from build123d import *

# Parameters (mm, degrees)
F1_DEPTH = 26
F3_DEPTH = 7
F4_R     = 5
F5_R     = 2.5


with BuildPart() as f1:
    # F0 (on Top) → F1 (new body)
    with BuildSketch(Plane.XY):
        Polygon((0, 30), (0, 0), (4, 0), (4, 26), (9.5, 26), (9.5, 0), (13.5, 0), (13.5, 15), (40.5, 20), (40.5, 120), (30.5, 120), (-5, 120), (-5, 110), (30.5, 110), (30.5, 30), align=None)
        with BuildLine():
            Line((4, 0), (0, 0))
            ThreePointArc((0, 0), (2, -2), (4, 0))
        make_face()
        with BuildLine():
            ThreePointArc((-5, 120), (-10, 115), (-5, 110))
            Line((-5, 110), (-5, 120))
        make_face()
        with BuildLine():
            Line((13.5, 0), (9.5, 0))
            ThreePointArc((9.5, 0), (11.5, -2), (13.5, 0))
        make_face()
    extrude(amount=F1_DEPTH)

    # F2 (on face) → F3 (cut)
    with BuildSketch(Plane(origin=(0, 0, 0), x_dir=(1, 0, 0), z_dir=(0, 0, -1))):
        with BuildLine():
            Line((13.5, -30), (30.5, -30))
            Line((30.5, -30), (30.5, -110))
            Line((30.5, -110), (-5, -110))
            ThreePointArc((-5, -110), (-10, -115), (-5, -120))
            Line((-5, -120), (13.5, -120))
            Line((13.5, -120), (40.5, -120))
            Line((40.5, -120), (40.5, -20))
            Line((40.5, -20), (13.5, -15))
            Line((13.5, -15), (13.5, -30))
        make_face()
    extrude(amount=-F3_DEPTH, mode=Mode.SUBTRACT)

    # F4
    f4_edges = [f1.edges().sort_by_distance(p)[0] for p in [
        (40.5, 120, 16.5),
        (30.5, 110, 16.5),
        (30.5, 30, 16.5),
        (40.5, 20, 16.5),
    ]]
    fillet(f4_edges, radius=F4_R)

    # F5
    f5_edges = [f1.edges().sort_by_distance(p)[0] for p in [
        (0, 30, 13),
        (4, 26, 13),
        (9.5, 26, 13),
        (13.5, 15, 16.5),
        (13.5, 30, 3.5),
    ]]
    fillet(f5_edges, radius=F5_R)


solid = f1.part
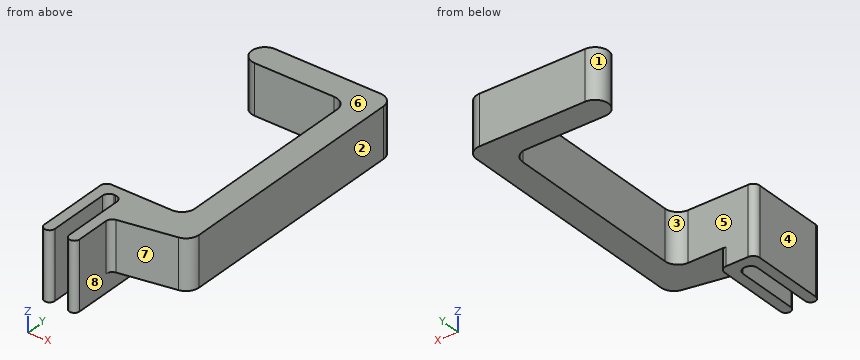
Input: part model. Units: mm. Frame: model coordinates. Face numbers are marked on the shaded views. A direction names the side the tool comes from. Coordinates: 2 decimals unless noted, no trailing zeros. Loops run counter-clockwise (first coordinate to the right, second up) from the corner with the lowest first, then second, coordinate; pieces in that order, holes last.
(1) Section C-C on x = 20.5. Return the cut outline in (y, z), then the cut area to 3 significant figures.
(2) Section D-D on y = 59.5. Return the cut outline in (x, z), then the cut area to 3 significant figures.
(3) First-contact query: pin 1 Ø12 at (y, z) = (17, 14) entering from +X; pin 2 Ø9.5 at (y, z) = (74, 14) entering from -X; pin 3 Ø4 at (x, z) = (34, 8.5) entering from -Y. Flat tips, straight axial feed; report the tip coordinate or a pass-through.
(4) Section B-B on z = 11.5. Return the cut outline in (x, y), then the cut area to 3 significant figures.
(5) Set-up query: the marked faces 4, 5, 6, 7 and 8. Return all of +Z, -Z, +X, -X, +Y, -Y with unobstructed straight access to the full face (end or side cutting, diameter ignored); none if empty.
(6) Pull-direction query (Y, two-part tool) for the marked faces 1, 2 and 3; classes: released by +Y, released by -Y, zero draft, split by the parting line, or undercut.
(7) Section A-A on y = 8. Return the cut outline in (x, z), then the cut area to 3 significant figures.
(8) Material intervals for probe 1 along X at (y, z) = (6, 25); probe 2 along Z at (x, y) = (33, 94); probe 3 along Y at (x, z) = (18, 17.5), sorted ascending.
Data:
1. outline: (16.3, 7) - (30, 7) - (30, 26) - (16.3, 26) - close; (110, 7) - (120, 7) - (120, 26) - (110, 26) - close
1. area: 450 mm2
2. outline: (30.5, 7) - (40.5, 7) - (40.5, 26) - (30.5, 26) - close
2. area: 190 mm2
3. pin 1: stops at x = 40.36
3. pin 2: stops at x = 30.5
3. pin 3: stops at y = 18.43
4. outline: (-5, 110) - (25.5, 110) arc R5 cw to (30.5, 105) - (30.5, 35) arc R5 cw to (25.5, 30) - (2.5, 30) arc R2.5 ccw to (0, 27.5) - (0, 0) arc R2 ccw to (4, 0) - (4, 23.5) arc R2.5 cw to (6.5, 26) - (7, 26) arc R2.5 cw to (9.5, 23.5) - (9.5, 0) arc R2 ccw to (13.5, 0) - (13.5, 12.92) arc R2.5 cw to (15.54, 15.38) - (36.41, 19.24) arc R5 ccw to (40.5, 24.16) - (40.5, 115) arc R5 ccw to (35.5, 120) - (-5, 120) arc R5 ccw to start
4. area: 1,910 mm2
5. face 4: +Z, -Z, -X, -Y
5. face 5: +Z, -Z, -X
5. face 6: +Z, +X, -X, +Y, -Y
5. face 7: +Z, -Z, +X, -Y
5. face 8: -Z, +X, -Y
6. face 1: split by the parting line
6. face 2: zero draft
6. face 3: undercut
7. outline: (0, 0) - (4, 0) - (4, 26) - (0, 26) - close; (9.5, 0) - (13.5, 0) - (13.5, 26) - (9.5, 26) - close
7. area: 208 mm2
8. probe 1: x = 0 to 4, 9.5 to 13.5
8. probe 2: z = 7 to 26
8. probe 3: y = 15.83 to 30, 110 to 120
